Design review of the part built by this model. Coordinates are the model's own, in mm. A direction names the side the tool comes from. Give positions to 0.01 mm unless a question says otherwise; leave off trailing zeros. Use a Markdown table: item, result. Add a question column.
(1) Add section A-A, the plane z = 0. State how many separate pieces and enclosed holes the cut face has, then the cut area to 3 significant figures.
(2) Insertion check: pin 1 Ø4 at (y, z) = (7, -1) entering from -X; pin 2 Ø3 at (y, z) = (4.5, -42) entering from -X; pin 3 Ø1 at (x, y) = (-41.5, 3) entering from +Z; pin 4 Ø3 at (x, z) = (-31.82, 31.82) entering from -Y. Each pin has a flat end and moves straight along its axis. Give the tip position at first contact, or say it passes through.
(3) For faces 4 (the face through (-30, 9, -37)), 5 (the face through (42.56, 4.93, -0.54)), list the 3-axis set-ups (+Z, -Z, +X, -X, +Y, -Y) from which the entire face can be reached by the end or side of a thin tool; tool diameter is ignored.
(4) For probe 1 along Z at (x, y) = (-30.5, 8.75); probe 2 along Z at (x, y) = (23, 9.25); probe 3 along Z at (x, y) = (17, 2), list the stretches that pass through material, from the lowest coordinate up.
(5) Draft analysis for pull direction X (two halves, no side actions). For faces 1 (the face through (-56.133, 4.93, -12.465)), 2 (the face through (44, 10, 16)), 3 (the face through (-36.7, 9.51, 30.74)), state which applies: pulls with the +X half, pulls with the -X half, needs draft (parallel to the pull), parting line crosses it, or undercut.
```python
from build123d import *

# Parameters (mm, degrees)
SKETCH1_R           = 57.5
SKETCH1_R_2         = 1.75
SKETCH1_R_3         = 26.1
SKETCH1_R_4         = 2.5
BOSS_EXTRUDE1_DEPTH = 10
SKETCH2_R           = 7
SKETCH2_R_2         = 5
CUT_EXTRUDE1_DEPTH  = 1


with BuildPart() as part:
    # Sketch1 → Boss-Extrude1 (new body)
    with BuildSketch(Plane(origin=(0, 0, 0), x_dir=(1, 0, 0), z_dir=(0, 1, 0))):
        with Locations(Location((0, 0, 0), (0, 0, 270))):
            Circle(SKETCH1_R)
        with Locations(Location((-10.534877389, 52.962405142, 0), (0, 0, 270))):
            Circle(SKETCH1_R_2, mode=Mode.SUBTRACT)
        with Locations(Location((10.534877389, 52.962405142, 0), (0, 0, 270))):
            Circle(SKETCH1_R_2, mode=Mode.SUBTRACT)
        with Locations(Location((30.000792583, 44.899359064, 0), (0, 0, 270))):
            Circle(SKETCH1_R_2, mode=Mode.SUBTRACT)
        with Locations(Location((44.899359064, 30.000792583, 0), (0, 0, 270))):
            Circle(SKETCH1_R_2, mode=Mode.SUBTRACT)
        with Locations(Location((52.962405142, 10.534877389, 0), (0, 0, 270))):
            Circle(SKETCH1_R_2, mode=Mode.SUBTRACT)
        with Locations(Location((52.962405142, -10.534877389, 0), (0, 0, 270))):
            Circle(SKETCH1_R_2, mode=Mode.SUBTRACT)
        with Locations(Location((44.899359064, -30.000792583, 0), (0, 0, 270))):
            Circle(SKETCH1_R_2, mode=Mode.SUBTRACT)
        with Locations(Location((30.000792583, -44.899359064, 0), (0, 0, 270))):
            Circle(SKETCH1_R_2, mode=Mode.SUBTRACT)
        with Locations(Location((10.534877389, -52.962405142, 0), (0, 0, 270))):
            Circle(SKETCH1_R_2, mode=Mode.SUBTRACT)
        with Locations(Location((-10.534877389, -52.962405142, 0), (0, 0, 270))):
            Circle(SKETCH1_R_2, mode=Mode.SUBTRACT)
        with Locations(Location((-30.000792583, -44.899359064, 0), (0, 0, 270))):
            Circle(SKETCH1_R_2, mode=Mode.SUBTRACT)
        with Locations(Location((-44.899359064, -30.000792583, 0), (0, 0, 270))):
            Circle(SKETCH1_R_2, mode=Mode.SUBTRACT)
        with Locations(Location((0, 0, 0), (0, 0, 270))):
            Circle(SKETCH1_R_3, mode=Mode.SUBTRACT)
        with Locations(Location((0, 45, 0), (0, 0, 270))):
            Circle(SKETCH1_R_4, mode=Mode.SUBTRACT)
        with Locations(Location((17.220754456, 41.574578963, 0), (0, 0, 270))):
            Circle(SKETCH1_R_4, mode=Mode.SUBTRACT)
        with Locations(Location((31.819805153, 31.819805153, 0), (0, 0, 270))):
            Circle(SKETCH1_R_4, mode=Mode.SUBTRACT)
        with Locations(Location((41.574578963, 17.220754456, 0), (0, 0, 270))):
            Circle(SKETCH1_R_4, mode=Mode.SUBTRACT)
        with Locations(Location((45, 0, 0), (0, 0, 270))):
            Circle(SKETCH1_R_4, mode=Mode.SUBTRACT)
        with Locations(Location((41.574578963, -17.220754456, 0), (0, 0, 270))):
            Circle(SKETCH1_R_4, mode=Mode.SUBTRACT)
        with Locations(Location((31.819805153, -31.819805153, 0), (0, 0, 270))):
            Circle(SKETCH1_R_4, mode=Mode.SUBTRACT)
        with Locations(Location((17.220754456, -41.574578963, 0), (0, 0, 270))):
            Circle(SKETCH1_R_4, mode=Mode.SUBTRACT)
        with Locations(Location((0, -45, 0), (0, 0, 270))):
            Circle(SKETCH1_R_4, mode=Mode.SUBTRACT)
        with Locations(Location((-17.220754456, -41.574578963, 0), (0, 0, 270))):
            Circle(SKETCH1_R_4, mode=Mode.SUBTRACT)
        with Locations(Location((-31.819805153, -31.819805153, 0), (0, 0, 270))):
            Circle(SKETCH1_R_4, mode=Mode.SUBTRACT)
        with Locations(Location((-41.574578963, -17.220754456, 0), (0, 0, 270))):
            Circle(SKETCH1_R_4, mode=Mode.SUBTRACT)
        with Locations(Location((-45, 0, 0), (0, 0, 270))):
            Circle(SKETCH1_R_4, mode=Mode.SUBTRACT)
        with Locations(Location((-41.574578963, 17.220754456, 0), (0, 0, 270))):
            Circle(SKETCH1_R_4, mode=Mode.SUBTRACT)
        with Locations(Location((-31.819805153, 31.819805153, 0), (0, 0, 270))):
            Circle(SKETCH1_R_4, mode=Mode.SUBTRACT)
        with Locations(Location((-17.220754456, 41.574578963, 0), (0, 0, 270))):
            Circle(SKETCH1_R_4, mode=Mode.SUBTRACT)
        with Locations(Location((-52.962405142, -10.534877389, 0), (0, 0, 270))):
            Circle(SKETCH1_R_2, mode=Mode.SUBTRACT)
        with Locations(Location((-52.962405142, 10.534877389, 0), (0, 0, 270))):
            Circle(SKETCH1_R_2, mode=Mode.SUBTRACT)
        with Locations(Location((-44.899359064, 30.000792583, 0), (0, 0, 270))):
            Circle(SKETCH1_R_2, mode=Mode.SUBTRACT)
        with Locations(Location((-30.000792583, 44.899359064, 0), (0, 0, 270))):
            Circle(SKETCH1_R_2, mode=Mode.SUBTRACT)
    extrude(amount=BOSS_EXTRUDE1_DEPTH)

    # Sketch2 → Cut-Extrude1 (cut)
    # profile 1 of 16: a face of its own
    with BuildSketch(Plane(origin=(0, 10, 0), x_dir=(1, 0, 0), z_dir=(0, 1, 0))):
        with Locations(Location((0, 45, 0), (0, 0, 270))):
            Circle(SKETCH2_R)
        with Locations(Location((0, 45, 0), (0, 0, 270))):
            Circle(SKETCH2_R_2, mode=Mode.SUBTRACT)
    # profile 2 of 16: a face of its own
    with BuildSketch(Plane(origin=(0, 10, 0), x_dir=(1, 0, 0), z_dir=(0, 1, 0))):
        with Locations(Location((17.220754456, 41.574578963, 0), (0, 0, 270))):
            Circle(SKETCH2_R)
        with Locations(Location((17.220754456, 41.574578963, 0), (0, 0, 270))):
            Circle(SKETCH2_R_2, mode=Mode.SUBTRACT)
    # profile 3 of 16: a face of its own
    with BuildSketch(Plane(origin=(0, 10, 0), x_dir=(1, 0, 0), z_dir=(0, 1, 0))):
        with Locations(Location((31.819805153, 31.819805153, 0), (0, 0, 270))):
            Circle(SKETCH2_R)
        with Locations(Location((31.819805153, 31.819805153, 0), (0, 0, 270))):
            Circle(SKETCH2_R_2, mode=Mode.SUBTRACT)
    # profile 4 of 16: a face of its own
    with BuildSketch(Plane(origin=(0, 10, 0), x_dir=(1, 0, 0), z_dir=(0, 1, 0))):
        with Locations(Location((41.574578963, 17.220754456, 0), (0, 0, 270))):
            Circle(SKETCH2_R)
        with Locations(Location((41.574578963, 17.220754456, 0), (0, 0, 270))):
            Circle(SKETCH2_R_2, mode=Mode.SUBTRACT)
    # profile 5 of 16: a face of its own
    with BuildSketch(Plane(origin=(0, 10, 0), x_dir=(1, 0, 0), z_dir=(0, 1, 0))):
        with Locations(Location((45, 0, 0), (0, 0, 270))):
            Circle(SKETCH2_R)
        with Locations(Location((45, 0, 0), (0, 0, 270))):
            Circle(SKETCH2_R_2, mode=Mode.SUBTRACT)
    # profile 6 of 16: a face of its own
    with BuildSketch(Plane(origin=(0, 10, 0), x_dir=(1, 0, 0), z_dir=(0, 1, 0))):
        with Locations(Location((41.574578963, -17.220754456, 0), (0, 0, 270))):
            Circle(SKETCH2_R)
        with Locations(Location((41.574578963, -17.220754456, 0), (0, 0, 270))):
            Circle(SKETCH2_R_2, mode=Mode.SUBTRACT)
    # profile 7 of 16: a face of its own
    with BuildSketch(Plane(origin=(0, 10, 0), x_dir=(1, 0, 0), z_dir=(0, 1, 0))):
        with Locations(Location((31.819805153, -31.819805153, 0), (0, 0, 270))):
            Circle(SKETCH2_R)
        with Locations(Location((31.819805153, -31.819805153, 0), (0, 0, 270))):
            Circle(SKETCH2_R_2, mode=Mode.SUBTRACT)
    # profile 8 of 16: a face of its own
    with BuildSketch(Plane(origin=(0, 10, 0), x_dir=(1, 0, 0), z_dir=(0, 1, 0))):
        with Locations(Location((17.220754456, -41.574578963, 0), (0, 0, 270))):
            Circle(SKETCH2_R)
        with Locations(Location((17.220754456, -41.574578963, 0), (0, 0, 270))):
            Circle(SKETCH2_R_2, mode=Mode.SUBTRACT)
    # profile 9 of 16: a face of its own
    with BuildSketch(Plane(origin=(0, 10, 0), x_dir=(1, 0, 0), z_dir=(0, 1, 0))):
        with Locations(Location((0, -45, 0), (0, 0, 270))):
            Circle(SKETCH2_R)
        with Locations(Location((0, -45, 0), (0, 0, 270))):
            Circle(SKETCH2_R_2, mode=Mode.SUBTRACT)
    # profile 10 of 16: a face of its own
    with BuildSketch(Plane(origin=(0, 10, 0), x_dir=(1, 0, 0), z_dir=(0, 1, 0))):
        with Locations(Location((-17.220754456, -41.574578963, 0), (0, 0, 270))):
            Circle(SKETCH2_R)
        with Locations(Location((-17.220754456, -41.574578963, 0), (0, 0, 270))):
            Circle(SKETCH2_R_2, mode=Mode.SUBTRACT)
    # profile 11 of 16: a face of its own
    with BuildSketch(Plane(origin=(0, 10, 0), x_dir=(1, 0, 0), z_dir=(0, 1, 0))):
        with Locations(Location((-31.819805153, -31.819805153, 0), (0, 0, 270))):
            Circle(SKETCH2_R)
        with Locations(Location((-31.819805153, -31.819805153, 0), (0, 0, 270))):
            Circle(SKETCH2_R_2, mode=Mode.SUBTRACT)
    # profile 12 of 16: a face of its own
    with BuildSketch(Plane(origin=(0, 10, 0), x_dir=(1, 0, 0), z_dir=(0, 1, 0))):
        with Locations(Location((-41.574578963, -17.220754456, 0), (0, 0, 270))):
            Circle(SKETCH2_R)
        with Locations(Location((-41.574578963, -17.220754456, 0), (0, 0, 270))):
            Circle(SKETCH2_R_2, mode=Mode.SUBTRACT)
    # profile 13 of 16: a face of its own
    with BuildSketch(Plane(origin=(0, 10, 0), x_dir=(1, 0, 0), z_dir=(0, 1, 0))):
        with Locations(Location((-45, 0, 0), (0, 0, 270))):
            Circle(SKETCH2_R)
        with Locations(Location((-45, 0, 0), (0, 0, 270))):
            Circle(SKETCH2_R_2, mode=Mode.SUBTRACT)
    # profile 14 of 16: a face of its own
    with BuildSketch(Plane(origin=(0, 10, 0), x_dir=(1, 0, 0), z_dir=(0, 1, 0))):
        with Locations(Location((-41.574578963, 17.220754456, 0), (0, 0, 270))):
            Circle(SKETCH2_R)
        with Locations(Location((-41.574578963, 17.220754456, 0), (0, 0, 270))):
            Circle(SKETCH2_R_2, mode=Mode.SUBTRACT)
    # profile 15 of 16: a face of its own
    with BuildSketch(Plane(origin=(0, 10, 0), x_dir=(1, 0, 0), z_dir=(0, 1, 0))):
        with Locations(Location((-31.819805153, 31.819805153, 0), (0, 0, 270))):
            Circle(SKETCH2_R)
        with Locations(Location((-31.819805153, 31.819805153, 0), (0, 0, 270))):
            Circle(SKETCH2_R_2, mode=Mode.SUBTRACT)
    # profile 16 of 16: a face of its own
    with BuildSketch(Plane(origin=(0, 10, 0), x_dir=(1, 0, 0), z_dir=(0, 1, 0))):
        with Locations(Location((-17.220754456, 41.574578963, 0), (0, 0, 270))):
            Circle(SKETCH2_R)
        with Locations(Location((-17.220754456, 41.574578963, 0), (0, 0, 270))):
            Circle(SKETCH2_R_2, mode=Mode.SUBTRACT)
    extrude(amount=-CUT_EXTRUDE1_DEPTH, mode=Mode.SUBTRACT)


solid = part.part
```
Established:
| question | item | result |
|---|---|---|
| 1 | separate pieces | 4 |
| 1 | enclosed holes | 0 |
| 1 | area | 520 mm^2 |
| 2 | pin 1 | x = -57.5 |
| 2 | pin 2 | x = -40.82 |
| 2 | pin 3 | z = 40.31 |
| 2 | pin 4 | through |
| 3 | face 4 | +Y |
| 3 | face 5 | +Y, -Y |
| 4 | probe 1 | -48.74 to -46.58, -43.22 to -33.94, -29.7 to 29.7, 33.94 to 43.22, 46.58 to 48.74 |
| 4 | probe 2 | -52.7 to -45.52, -37.62 to -12.34, 12.34 to 37.62, 45.52 to 52.7 |
| 4 | probe 3 | -54.93 to -44.06, -39.08 to -19.8, 19.8 to 39.08, 44.06 to 54.93 |
| 5 | face 1 | parting line crosses it |
| 5 | face 2 | needs draft |
| 5 | face 3 | undercut |
